Check sheet for the modelled part. Datum: model origin and axes. Units: mm. A direction names the side the tool comes from. Give positions to 0.01 mm unless a question says otherwise; leave off trailing zeros. Loops run counter-clockwise (first coordinate to the right, second up) from the corner with the lowest first, then second, coordinate; pieces in that order, holes last. Notation, with made-up numbers: (34, 59.5) -> (50, 59.5) arc R15 ccw to (50, 65.5) -> close; hole circle Ø10 at (72.5, 82.5). An arc over 180 degrees is marked (long way). Write each question's results on one line, items separated by ' | '. Start each with the question number.
1. Cross-section at C-C on x = 10. Record the boundary of the cut face in (y, z) (3 decimals), and give its area (3 significant figures).
2. Cross-section at D-D on y = 12.5. Record the boundary of the cut face in (x, z), and give its area (3 significant figures).
3. Gauge pin test, flat ends, axial feed: pin 1 Ø1 at (x, z) = (9, 1) entering from +Y; pin 2 Ø1.6 at (y, z) = (12.5, 21.65) entering from +X; pin 3 Ø1.4 at (x, z) = (7, -17.5) entering from +Y; pin 4 Ø6 at (x, z) = (2.5, 6) entering from -Y. Record the tip position at first contact, or that the pin passes through.
4. Material ranges on L1, parallel to Y at x = 3.4, z = 0 (3 decimals); L2, parallel to Y at x = 4.75, z = -21.5; L3, parallel to X at y = 20.5, z = 5.5, recorded low to high. Write a range as from..to.
5. Cross-section at A-A on y = -25. Record the boundary of the cut face in (x, z).
6. Cross-section at B-B on z = -15. Record the boundary of the cut face in (x, y).
7. Mould release check, pull along Y, two halves, no side actions. Record for faces 4 (the face through (2.47, -11.21, -21.82)), 5 (the face through (12.1, -9, -15)), 6 (the face through (8.7, 19.9, -0.1)): +Y half, -Y half, draft (parallel to the pull), parting line (faces both ways), or undercut.
8. Tool access check on faces 1 (the face through (5.2, -6.31, -20.03)), 2 (the face through (8.7, -15.59, 9)), 3 (the face through (8.7, 15.55, -8.98)). Record the directions out of +Z, -Z, +X, -X, +Y, -Y that give a thin tool (end or side, any length) a straight path to the whole face; none if there is none.
from build123d import *

# Parameters (mm, degrees)
SKIZZE2_R                        = 16.075
SCHNITT_LINEAR_AUSTRAGEN1_DEPTH  = 45.873823104344474
F_2_6_2_6_DURCHMESSER_BOHRUNG1_D = 2.6
KREISMUSTER1_COUNT               = 6
AUFSATZ_LINEAR_AUSTRAGEN1_DEPTH  = 6.7
VERRUNDUNG1_R                    = 0.5
KREISMUSTER2_START               = 5.4
KREISMUSTER2_DEPTH               = 6.7


# Read off the part's stored shape, not the designer's step: Kreismuster2
with BuildPart() as part:
    # Skizze1 → Rotation1 (revolve)
    with BuildSketch(Plane.XY, mode=Mode.PRIVATE) as rotation1_sk:
        Polygon((0, 0), (0, 31.5), (4.999999999999999, 31.5), (5.000000000000001, 20.999999999999996), (5.4, 21), (5.4, 0), align=None)
    revolve(rotation1_sk.sketch.rotate(Axis((0, 0, 0), (-1, 0, 0)), 90), axis=Axis((0, 0, 0), (-1, 0, 0)))

    # Skizze2 → Schnitt-Linear austragen1 (cut, through all)
    with BuildSketch(Plane.ZY):
        Circle(SKIZZE2_R)
    extrude(amount=-SCHNITT_LINEAR_AUSTRAGEN1_DEPTH, mode=Mode.SUBTRACT)

    # Ø2.6 (2.6) Durchmesser Bohrung1 (through all)
    with Locations(Plane(origin=(5, 0, 0), x_dir=(0, 0, -1), z_dir=(1, 0, 0))):
        with Locations((0, 25)):
            f_2_6_2_6_durchmesser_bohrung1 = Hole(F_2_6_2_6_DURCHMESSER_BOHRUNG1_D / 2)

    # Kreismuster1: Ø2.6 (2.6) Durchmesser Bohrung1 ×6 about axis
    kreismuster1_axis = Axis((0, -7.2e-16, -2.984e-14), (1, 0, 0))
    for i in range(1, KREISMUSTER1_COUNT):
        add(f_2_6_2_6_durchmesser_bohrung1.rotate(kreismuster1_axis, i * 360 / KREISMUSTER1_COUNT), mode=Mode.SUBTRACT)

    # Skizze5 → Aufsatz-Linear austragen1 (add)
    with BuildSketch(Plane(origin=(5.4, 0, 0), x_dir=(0, 0, -1), z_dir=(1, 0, 0))):
        with BuildLine():
            Line((-9.950000000000019, 17.233905535310317), (-8.037500000000017, 13.921358365834841))
            ThreePointArc((-8.037500000000017, 13.921358365834841), (9.8e-16, 16.075), (8.037500000000014, 13.921358365834843))
            Line((8.037500000000014, 13.921358365834843), (9.950000000000017, 17.233905535310317))
            ThreePointArc((9.950000000000017, 17.233905535310317), (1.22e-15, 19.9), (-9.950000000000019, 17.233905535310317))
        make_face()
    extrude(amount=AUFSATZ_LINEAR_AUSTRAGEN1_DEPTH)

    # Verrundung1
    verrundung1_edges = [part.edges().sort_by_distance(p)[0] for p in [
        (8.75, 17.233905535310317, -9.950000000000015),
        (8.75, 17.23390553531032, 9.950000000000017),
        (8.75, 13.921358365834843, 8.03750000000002),
        (8.75, 13.921358365834845, -8.037500000000014),
    ]]
    fillet(verrundung1_edges, radius=VERRUNDUNG1_R)

    # Kreismuster2 outline → Kreismuster2 (add)
    with BuildSketch(Plane.YZ.offset(KREISMUSTER2_START)):
        with BuildLine():
            ThreePointArc((-13.672564308, 8.453792655), (-8.0375, 13.921358366), (-0.484917044, 16.067684353))
            ThreePointArc((-0.484917044, 16.067684353), (-0.1411536, 16.219276879), (0, 16.567456805))
            Line((0, 16.567456805), (0, 19.393555631))
            ThreePointArc((0, 19.393555631), (-0.151032451, 19.751636138), (-0.512886598, 19.893389539))
            ThreePointArc((-0.512886598, 19.893389539), (-9.95, 17.233905535), (-16.971737409, 10.390867592))
            ThreePointArc((-16.971737409, 10.390867592), (-17.029902436, 10.006616008), (-16.795311846, 9.696777815))
            Line((-16.795311846, 9.696777815), (-14.34783847, 8.283728403))
            ThreePointArc((-14.34783847, 8.283728403), (-13.975729009, 8.231881043), (-13.672564308, 8.453792655))
        make_face()
        with BuildLine():
            ThreePointArc((0, -16.567456805), (-0.1411536, -16.219276879), (-0.484917044, -16.067684353))
            ThreePointArc((-0.484917044, -16.067684353), (-8.0375, -13.921358366), (-13.672564308, -8.453792655))
            ThreePointArc((-13.672564308, -8.453792655), (-13.975729009, -8.231881043), (-14.34783847, -8.283728403))
            Line((-14.34783847, -8.283728403), (-16.795311846, -9.696777815))
            ThreePointArc((-16.795311846, -9.696777815), (-17.029902436, -10.006616008), (-16.971737409, -10.390867592))
            ThreePointArc((-16.971737409, -10.390867592), (-9.95, -17.233905535), (-0.512886598, -19.893389539))
            ThreePointArc((-0.512886598, -19.893389539), (-0.151032451, -19.751636138), (0, -19.393555631))
            Line((0, -19.393555631), (0, -16.567456805))
        make_face()
    extrude(amount=KREISMUSTER2_DEPTH)


solid = part.part
Geometry says:
1) outline: (-16.972, -10.391) arc R19.9 ccw to (-0.513, -19.893) arc R0.5 ccw to (0, -19.394) -> (0, -16.567) arc R0.5 ccw to (-0.485, -16.068) arc R16.075 cw to (-13.673, -8.454) arc R0.5 ccw to (-14.348, -8.284) -> (-16.795, -9.697) arc R0.5 ccw to start; (-16.972, 10.391) arc R0.5 ccw to (-16.795, 9.697) -> (-14.348, 8.284) arc R0.5 ccw to (-13.673, 8.454) arc R16.075 cw to (-0.485, 16.068) arc R0.5 ccw to (0, 16.567) -> (0, 19.394) arc R0.5 ccw to (-0.513, 19.893) arc R19.9 ccw to start; (14.157, -7.614) arc R0.5 ccw to (14.348, -8.284) -> (16.795, -9.697) arc R0.5 ccw to (17.485, -9.503) arc R19.9 ccw to (17.485, 9.503) arc R0.5 ccw to (16.795, 9.697) -> (14.348, 8.284) arc R0.5 ccw to (14.157, 7.614) arc R16.075 cw to start | area: 216 mm^2
2) outline: (0, -28.91) -> (5, -28.91) -> (5, -22.95) -> (0, -22.95) -> close; (0, -20.35) -> (5, -20.35) -> (5, -16.87) -> (5.4, -16.87) -> (5.4, -10.11) -> (0, -10.11) -> close; (0, 10.11) -> (5.4, 10.11) -> (5.4, 16.87) -> (5, 16.87) -> (5, 20.35) -> (0, 20.35) -> close; (0, 22.95) -> (5, 22.95) -> (5, 28.91) -> (0, 28.91) -> close | area: 167 mm^2
3) pin 1: y = 19.89 | pin 2: through | pin 3: y = 0 | pin 4: y = -31.36
4) L1: -31.5..-26.3, -23.7..-16.075, 16.075..23.7, 26.3..31.5 | L2: -23.02..-13.79, -11.21..11.21, 13.79..23.02 | L3: 0..5
5) outline: (0, -19.16) -> (5, -19.16) -> (5, -1.3) -> (0, -1.3) -> close; (0, 1.3) -> (5, 1.3) -> (5, 19.16) -> (0, 19.16) -> close
6) outline: (0, -27.7) -> (5, -27.7) -> (5, -14.7) -> (5.4, -14.7) -> (5.4, -13.08) -> (12.1, -13.08) -> (12.1, -5.78) -> (0, -5.78) -> close; (0, 5.78) -> (5.4, 5.78) -> (5.4, 14.7) -> (5, 14.7) -> (5, 27.7) -> (0, 27.7) -> close
7) face 4: undercut | face 5: draft | face 6: +Y half
8) face 1: +X | face 2: +X, -Y | face 3: -Z, +X
